Drawing for the job (mm, zero at the part's lowest x, y, z). Give positions to 0.01 mm unless a question says otherwise; leave off trailing zeros. Write each loop counter-clockwise with the first axis right and the second up, starting at its lowest first coordinate (ties: lowest second). Pieces come first, ordered by that corner, then holes. Notation, with made-up numbers: (-39.75, -38.5) - (-13.75, -38.5) arc R7 ccw to (-13.75, -26.5) - close; hole circle Ø7 at (11, -20.5). An arc over 180 degrees is marked (long way). Write item = value, one per line. Start each with the question number.
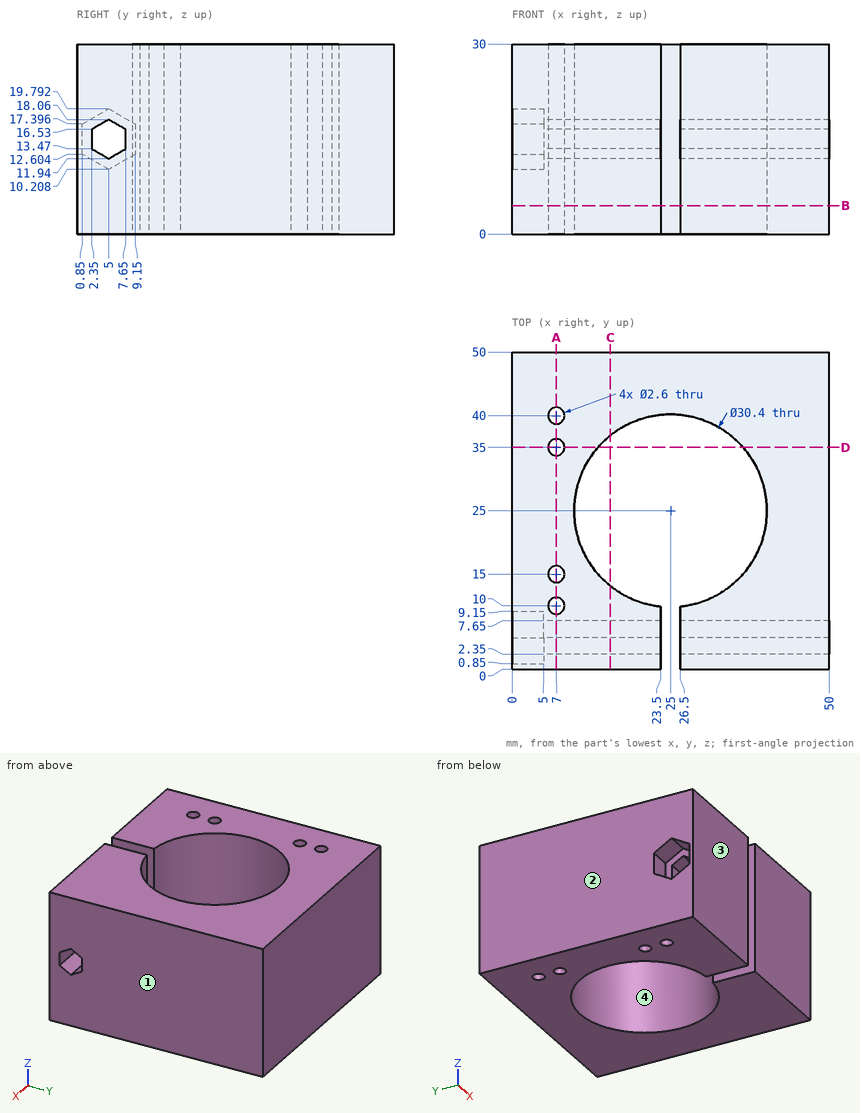
1. Cut at A-A (x = 7). Give the cut face in (y, z), then the cut area to 3 significant figures.
2. Cut at C-C (x = 15.5). Give the cut face in (y, z), then the cut area to 3 significant figures.
3. Wall check: line 1 along Y through (x, z) = (7, 24); line 2 along X through (y, z) = (25, 8); line 3 along Y through (x, z) = (25, 21). Give the ranges that are in metal, low to high.
4. Cut at B-B (z = 4.5). Give the cut face in (x, y), then the cut area to 3 significant figures.
5. Pin check, flat tip, straight feed: pin 1 Ø6.5 at (y, z) = (4.5, 14.5) entering from -X. Stop position of the tip, or through.
6. Cut at D-D (y = 35). Give the cut face in (x, z).
7. Mould opens along X. For the marked faces 1, 2, 3 and 4 say: +X half, -X half, draft (parallel to the pull), parting line (faces both ways), or undercut.
Output:
q1.outline = (0, 0) - (8.7, 0) - (8.7, 30) - (0, 30) - close; (11.3, 0) - (13.7, 0) - (13.7, 30) - (11.3, 30) - close; (16.3, 0) - (33.7, 0) - (33.7, 30) - (16.3, 30) - close; (36.3, 0) - (38.7, 0) - (38.7, 30) - (36.3, 30) - close; (41.3, 0) - (50, 0) - (50, 30) - (41.3, 30) - close; hole (2.35, 13.47) - (5, 11.94) - (7.65, 13.47) - (7.65, 16.53) - (5, 18.06) - (2.35, 16.53) - close
q1.area = 1,160 mm2
q2.outline = (0, 0) - (13.13, 0) - (13.13, 30) - (0, 30) - close; (36.87, 0) - (50, 0) - (50, 30) - (36.87, 30) - close; hole (2.35, 13.47) - (5, 11.94) - (7.65, 13.47) - (7.65, 16.53) - (5, 18.06) - (2.35, 16.53) - close
q2.area = 764 mm2
q3.line_1 = 0 to 8.7, 11.3 to 13.7, 16.3 to 33.7, 36.3 to 38.7, 41.3 to 50
q3.line_2 = 0 to 9.8, 40.2 to 50
q3.line_3 = 40.2 to 50
q4.outline = (0, 0) - (23.5, 0) - (23.5, 9.87) arc R15.2 cw (long way) to (26.5, 9.87) - (26.5, 0) - (50, 0) - (50, 50) - (0, 50) - close; hole circle Ø2.6 at (7, 10); hole circle Ø2.6 at (7, 15); hole circle Ø2.6 at (7, 35); hole circle Ø2.6 at (7, 40)
q4.area = 1,720 mm2
q5.pin_1 = 5
q6.outline = (0, 0) - (5.7, 0) - (5.7, 30) - (0, 30) - close; (8.3, 0) - (13.55, 0) - (13.55, 30) - (8.3, 30) - close; (36.45, 0) - (50, 0) - (50, 30) - (36.45, 30) - close
q7.face_1 = +X half
q7.face_2 = -X half
q7.face_3 = draft
q7.face_4 = undercut
